Design review of the part built by this model. Coordinates are the model's own, in mm. A direction names the side the tool comes from. Round coordinates to 2 decimals unless told otherwise and drop trailing zeros. Order: outer loops, then holes, each group sorted by start corner. A loop starts at its lowest first (then second) coordinate and runs counter-clockwise, first axis right, second up. Notation, with made-up numbers: M 11.5,81 L 50.5,81 A11 ccw 50.5,100 Z; hole C 86.5,58.25 d1. An arc over 180 degrees is marked long. Write each question's results on one line, items separated by ' | '. Start each with the question number.
Item 1: Clearance check with flat-ended pins moving along their axes: pin 1 (2 mm diameter, centred on x = 42, y = 12, fed in from +Z); pin 2 (2 mm diameter, centred on x = 3, z = 3, fed in from -Y); pin 3 (1.5 mm diameter, centred on y = 47.5, z = 3, fed in from -X). State where each tip first meets the part, or that it passes through.
Item 2: Machinability: for faces 5 (the flat face through (6, 30, 6)), 6 (the flat face through (147, 30, 5)), which of the approach directions +Z, -Z, +X, -X, +Y, -Y give a long, thin tool a straight path to every point of the face, cutting with its end or side? Answer none if there is none.
Item 3: Take a section at B-B, the plane x = 97. Write out the cut boundary in (y, z).
Item 4: Take a section at A-A, the plane y = 37.5. Write out the cut boundary in (x, z), plus the area to 3 significant figures.
Item 5: Wall thickness on line 1 (Y direction, x = 153, z = 3); line 2 (Z direction, x = 156.5, y = 12.5); line 3 (Z direction, x = 115, y = 30.5): over which ranges is each line inside the solid? List them lowest first. Write a range as [from, to].
Item 6: The part is to be moulded in two halves that separate along X. For faces 1 (the flat face through (0, 30, 3)), 2 (the flat face through (79, 30, 0)), 3 (the flat face through (14, 30, 4)), 4 (the flat face through (81, 30, 3)), say which applies: +X half, -X half, draft (parallel to the pull), parting line (faces both ways), or undercut.
Autodesk Inventor part; units mm, degrees
ref_plane "YZ Plane" through (0, 0, 0) normal (1, 0, 0) x (0, 1, 0)
ref_plane "XZ Plane" through (0, 0, 0) normal (0, 1, 0) x (-1, 0, 0)
ref_plane "XY Plane" through (0, 0, 0) normal (0, 0, 1) x (1, 0, 0)
sketch "Sketch1" plane through (0, 0, 0) normal (0, 0, 1) x (1, 0, 0)
  line L0 (0, 0) -> (160, 0)
  line L1 (160, 0) -> (160, 60)
  line L2 (160, 60) -> (0, 60)
  line L3 (0, 60) -> (0, 0)
  dimension "d0" = 160
  dimension "d1" = 60
extrude "Extrusion1" add sketch "Sketch1" along normal blind 6
sketch "Sketch2" plane through (0, 0, 0) normal (0, -1, 0) x (1, 0, 0)
  line L0 (3, 3) -> (157, 3) construction
  line L1 (160, 0) -> (0, 0) construction
  line L2 (0, 6) -> (160, 6) construction
  line L3 (160, 0) -> (160, 6) construction
  line L4 (0, 0) -> (0, 6) construction
  point P0 (0, 3)
  dimension "d4" = 3
  dimension "d5" = 6
  dimension "d6" = 3
  dimension "d7" = 3
hole "Hole1" at (3, 0, 3) at (157, 0, 3) direction (0, 1, 0) diameter 2.459 depth 8.8 tip angle 118
chamfer "Chamfer1" distance 0.3 angle 45 2 edges at (3, 0, 4.2295) (157, 0, 4.2295)
sketch "Sketch3" plane through (0, 60, 0) normal (0, 1, 0) x (1, 0, 0)
  line L0 (160, -6) -> (0, -6)
  line L1 (148, -6) -> (145, -3)
  line L2 (148, -6) -> (152.2426, -6) construction
  line L3 (145, -3) -> (15, -3)
  line L4 (160, 0) -> (0, 0)
  line L5 (15, -3) -> (12, -6)
  line L6 (12, -6) -> (148, -6)
  line L7 (160, 0) -> (160, -6)
  line L8 (0, 0) -> (0, -6)
  point P0 (12, -6)
  point P1 (0, -3)
  dimension "d18" = 135
  dimension "d19" = 3
  dimension "d22" = 15
  dimension "d23" = 130
  dimension "d24" = 15
extrude "Extrusion2" cut sketch "Sketch3" against normal through all contours L0 L5 L3 L1
sketch "Sketch6" plane through (160, 0, 0) normal (1, 0, 0) x (0, 0, -1)
  line L0 (-3, 60) -> (-3, 0)
  circle A0 centre (-3, 12.5) radius 1.5
  circle A1 centre (-3, 47.5) radius 1.5
  line L1 (0, 0) -> (-6, 0)
  line L2 (0, 60) -> (-6, 60)
  dimension "d34" = 3
  dimension "d35" = 3
  dimension "d36" = 35
  dimension "d37" = 12.5
  dimension "d38" = 60
hole "Hole2" at (160, 12.5, 3) at (160, 47.5, 3) direction (-1, 0, 0) diameter 2.459 depth 8.8 tip angle 118
sketch "Sketch7" plane through (0, 0, 0) normal (-1, 0, 0) x (0, 0, 1)
  line L0 (3, 60) -> (3, 0)
  circle A0 centre (3, 12.5) radius 1.5
  circle A1 centre (3, 47.5) radius 1.5
  line L1 (0, 60) -> (6, 60)
  line L2 (0, 0) -> (6, 0)
  dimension "d46" = 3
  dimension "d47" = 3
  dimension "d48" = 35
  dimension "d49" = 60
  dimension "d50" = 12.5
hole "Hole3" at (0, 47.5, 3) at (0, 12.5, 3) direction (1, 0, 0) diameter 2.459 depth 8.8 tip angle 118
equation "\"d4\" = 0.5 * d5"
equation "\"d22\" = d24"
equation "\"d37\" = -0.5 * d36 + 0.5 * d38"
equation "\"d50\" = -0.5 * d48 + 0.5 * d49"
properties part number "Prawa ściana"
Results list:
1) pin 1: z = 3 | pin 2: y = 8.94 | pin 3: x = 9.09
2) face 5: +Z, +X, -X, +Y, -Y | face 6: +Z, +Y, -Y
3) outline: M 0,0 L 60,0 L 60,3 L 0,3 Z
4) outline: M 0,0 L 160,0 L 160,6 L 148,6 L 145,3 L 15,3 L 12,6 L 0,6 Z | area: 561 mm²
5) line 1: [0, 11.27], [13.73, 46.27], [48.73, 60] | line 2: [0, 1.77], [4.23, 6] | line 3: [0, 3]
6) face 1: -X half | face 2: draft | face 3: undercut | face 4: undercut
